Work out the finished part from the listing and answer in its coordinate system (mm). A direction names the side the tool comes from. Give positions to 0.01 mm unless a question says otherwise; leave off trailing zeros. Loops run counter-clockwise (first coordinate to the right, second up) from the corner with the lowest first, then second, coordinate; pieces in that order, holes last. Notation, with made-up numbers: M 29,-22 L 84,-22 A35 cw 84,13 Z; hole C 66.25,52 d3. An arc over 180 degrees is marked long. Write item = value, one per line. Start each with the question number.
1. A flat-ended cylindrical pin translates along its axis: pin 1 Ø1.9 at (x, y) = (4.5, -10.5) entering from +Z. Find the tip coordinate at first contact, or state that the pin passes through.
2. For faces 1 (the face through (-4, -12.7, 17)), 2 (the face through (304.006, -9, 0)), determine the directions among +Z, -Z, +X, -X, +Y, -Y from which every point of the face is accessible in a straight line to the end or side of a thin tool.
3. Consider L1, parallel to Y at x = -97.5, z = 16; L2, parallel to Z at x = -87, y = -7 (1 decimal); L3, parallel to Y at x = -191, z = 20 (3 decimals). Determine where each line is inside the solid, lowest interval first. Write a range as [from, to].
4. Section B-B on y = -9.5 is taken. Determine the outline of the cut face in (x, z) (1 decimal), plus the area to 3 significant figures.
5. The mould has two halves that part along Y. Classify faces 3 (the face through (-4, -6.35, 17)), 4 (the face through (-304.006, -9, 0)), 5 (the face through (-4, -19.05, -1)): released by +Y, released by -Y, zero draft, split by the parting line, or undercut.
```python
from build123d import *

# Parameters (mm, degrees)
F0_W     = 608.0125
F0_H     = 44.45
F1_DEPTH = 19.05
F2_W     = 6.35
F2_H     = 11.1125
F3_DEPTH = 608.0135
F4_SIZE2 = 3.175
F4_SIZE  = 1.5875


with BuildPart() as f1:
    # F0 (on Front) → F1 (new body)
    with BuildSketch(Plane.XZ):
        Rectangle(F0_W, F0_H)
    extrude(amount=F1_DEPTH)

    # F2 (on face) → F3 (cut, through all)
    with BuildSketch(Plane(origin=(-304.00625, 0, 0), x_dir=(0, -1, 0), z_dir=(-1, 0, 0))):
        with Locations((9.525, 16.66875)):
            Rectangle(F2_W, F2_H)
    extrude(amount=-F3_DEPTH, mode=Mode.SUBTRACT)

    # F4
    f4_edges = [f1.edges().sort_by_distance(p)[0] for p in [
        (0, -19.05, 22.225),
    ]]
    chamfer(f4_edges, length=F4_SIZE, length2=F4_SIZE2)


solid = f1.part
```
Verdict:
q1.pin_1 = 11.11
q2.face_1 = +Z, +X, -X
q2.face_2 = +Z, -Z, +X, +Y, -Y
q3.L1 = [-19.05, -12.7], [-6.35, 0]
q3.L2 = [-22.2, 11.1]
q3.L3 = [-18.575, -12.7], [-6.35, 0]
q4.outline = M -304,-22.2 L 304,-22.2 L 304,11.1 L -304,11.1 Z
q4.area = 20,300 mm2
q5.face_3 = undercut
q5.face_4 = zero draft
q5.face_5 = released by -Y
